Read the model definition and answer for the solid it produces. Units are mm, in the model's axes. Give positions to 0.01 mm unless a question says otherwise; leave off trailing zeros. Write each loop counter-clockwise with the first axis right and the second up, starting at its lowest first coordinate (ties: lowest second). Pieces come first, ordered by that corner, then holes. Notation, with made-up numbers: M 70.25,-17.5 L 116.25,-17.5 A24 ccw 116.25,-5.5 Z; hole C -1.75,-13 d5. An arc over 180 degrees is marked long. Answer as CSV lines item,"result". Start each with the question number.
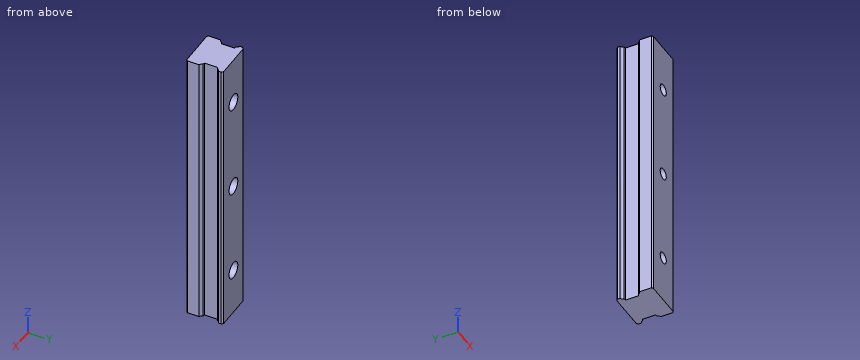
```python
from build123d import *

# Parameters (mm, degrees)
RESSALTO_EXTRUS_O1_DEPTH                             = 450
REBAIXO_PARA_PARAFUSO_DE_CABE_A_SEXTAVAD_D           = 18
REBAIXO_PARA_PARAFUSO_DE_CABE_A_SEXTAVAD_DEPTH       = 58
REBAIXO_PARA_PARAFUSO_DE_CABE_A_SEXTAVAD_CBORE_D     = 26
REBAIXO_PARA_PARAFUSO_DE_CABE_A_SEXTAVAD_CBORE_DEPTH = 25
CHANFRO1_SIZE2                                       = 2.500287455
CHANFRO1_SIZE                                        = 2.500257245
CHANFRO2_SIZE2                                       = 2.500423779
CHANFRO2_SIZE                                        = 2.500287455
CHANFRO3_SIZE                                        = 2


with BuildPart() as part:
    # Esboço1 → Ressalto-extrusão1 (new body)
    with BuildSketch(Plane.XY):
        with BuildLine():
            Line((-31.5, 20.527298986), (-31.5, 0))
            Line((-31.5, 0), (31.5, 0))
            Line((31.5, 0), (31.5, 20.527298986))
            ThreePointArc((31.5, 20.527298986), (28.900076881, 22.150342104), (27.397266061, 24.82156445))
            Line((27.397266061, 24.82156445), (24.5, 25.597882749))
            Line((24.5, 25.597882749), (24.5, 46.397686197))
            Line((24.5, 46.397686197), (27.397119712, 47.17387922))
            ThreePointArc((27.397119712, 47.17387922), (28.898613337, 49.848990738), (31.5, 51.474872705))
            Line((31.5, 51.474872705), (31.5, 58))
            Line((31.5, 58), (-31.5, 58))
            Line((-31.5, 58), (-31.5, 51.474872705))
            ThreePointArc((-31.5, 51.474872705), (-28.899411057, 49.849685923), (-27.397802135, 47.175837466))
            Line((-27.397802135, 47.175837466), (-24.5, 46.399706372))
            Line((-24.5, 46.399706372), (-24.5, 25.596973237))
            Line((-24.5, 25.596973237), (-27.397939574, 24.823365186))
            ThreePointArc((-27.397939574, 24.823365186), (-28.900095464, 22.151244343), (-31.5, 20.527298986))
        make_face()
    extrude(amount=RESSALTO_EXTRUS_O1_DEPTH)

    # Rebaixo para parafuso de cabeça sextavada de M161
    with Locations(Plane(origin=(0, 58, 0), x_dir=(1, 0, 0), z_dir=(0, 1, 0))):
        with Locations((0, -75), (0, -1425), (0, -1275), (0, -1125), (0, -975), (0, -825), (0, -675), (0, -525), (0, -375), (0, -225)):
            CounterBoreHole(REBAIXO_PARA_PARAFUSO_DE_CABE_A_SEXTAVAD_D / 2, REBAIXO_PARA_PARAFUSO_DE_CABE_A_SEXTAVAD_CBORE_D / 2, REBAIXO_PARA_PARAFUSO_DE_CABE_A_SEXTAVAD_CBORE_DEPTH, depth=REBAIXO_PARA_PARAFUSO_DE_CABE_A_SEXTAVAD_DEPTH)

    # Chanfro1
    chanfro1_edges = [part.edges().sort_by_distance(p)[0] for p in [
        (-31.5, 58, 225),
    ]]
    chamfer(chanfro1_edges, length=CHANFRO1_SIZE, length2=CHANFRO1_SIZE2)

    # Chanfro2
    chanfro2_edges = [part.edges().sort_by_distance(p)[0] for p in [
        (31.5, 58, 225),
    ]]
    chamfer(chanfro2_edges, length=CHANFRO2_SIZE, length2=CHANFRO2_SIZE2)

    # Chanfro3
    chanfro3_edges = [part.edges().sort_by_distance(p)[0] for p in [
        (31.5, 0, 225),
        (-31.5, 0, 225),
    ]]
    chamfer(chanfro3_edges, length=CHANFRO3_SIZE)


solid = part.part
```
1. Find section D-D on z = 313.5. Determine the outline of the cut face in (x, y), then the cut area to 3 significant figures.
2. Find the intervals of material crossed by line 1 (Z direction, x = 0, y = 40); line 2 (Z direction, x = 0, y = 11.5); line 3 (X direction, y = 44.25, z = 375), in increasing order. Write a range as [from, to].
3. Find section B-B on x = 0. Determine the outline of the cut face in (y, z).
4. Given pin 1 (4 mm diameter, centred on y = 30.5, z = 127.5, fed in from -X); pin 2 (14.5 mm diameter, centred on x = 0, z = 375, fed in from +Y); pin 3 (1 mm diameter, centred on y = 36, z = 312.5, fed in from +X), each flat-ended and moving along its own axis, determine where each tip first touches the part or whether it passes through.
5. Find section C-C on z = 375. Determine the outline of the cut face in (x, y), then the cut area to 3 significant figures.
6. Find section A-A on y = 11. Determine the outline of the cut face in (x, z), then the cut area to 3 significant figures.
Computed:
1,outline,"M -31.5,2 L -29.5,0 L 29.5,0 L 31.5,2 L 31.5,20.53 A6.19 cw 27.4,24.82 L 24.5,25.6 L 24.5,46.4 L 27.4,47.17 A6.19 cw 31.5,51.47 L 31.5,55.5 L 29,58 L -29,58 L -31.5,55.5 L -31.5,51.47 A6.19 cw -27.4,47.18 L -24.5,46.4 L -24.5,25.6 L -27.4,24.82 A6.19 cw -31.5,20.53 Z"
1,area,"3,290 mm^2"
2,line 1,"z = [0, 62], [88, 212], [238, 362], [388, 450]"
2,line 2,"z = [0, 66], [84, 216], [234, 366], [384, 450]"
2,line 3,"x = [-24.5, -13], [13, 24.5]"
3,outline,"M 0,0 L 58,0 L 58,62 L 33,62 L 33,66 L 0,66 Z; M 0,84 L 33,84 L 33,88 L 58,88 L 58,212 L 33,212 L 33,216 L 0,216 Z; M 0,234 L 33,234 L 33,238 L 58,238 L 58,362 L 33,362 L 33,366 L 0,366 Z; M 0,384 L 33,384 L 33,388 L 58,388 L 58,450 L 0,450 Z"
4,pin 1,"stops at x = -24.5"
4,pin 2,"passes through"
4,pin 3,"stops at x = 24.5"
5,outline,"M -31.5,2 L -29.5,0 L -9,0 L -9,33 L -13,33 L -13,58 L -29,58 L -31.5,55.5 L -31.5,51.47 A6.19 cw -27.4,47.18 L -24.5,46.4 L -24.5,25.6 L -27.4,24.82 A6.19 cw -31.5,20.53 Z; M 9,0 L 29.5,0 L 31.5,2 L 31.5,20.53 A6.19 cw 27.4,24.82 L 24.5,25.6 L 24.5,46.4 L 27.4,47.17 A6.19 cw 31.5,51.47 L 31.5,55.5 L 29,58 L 13,58 L 13,33 L 9,33 Z"
5,area,"2,040 mm^2"
6,outline,"M -31.5,0 L 31.5,0 L 31.5,450 L -31.5,450 Z; hole C 0,75 d18; hole C 0,225 d18; hole C 0,375 d18"
6,area,"27,600 mm^2"
